Input: part model. Units: mm. Frame: model coordinates. A direction names the side the tool comes from. Round coordinates to 2 decimals unless told otherwise and drop trailing zeros. Loops run counter-clockwise (first coordinate to the right, second up) from the corner with the lowest first, then second, coordinate; pieces in that order, holes last.
1) Section B-B, the plane z = 31. Return loops of the section in (x, y).
2) Access query for faces 5 (the face through (101, -7.5, 19)), 6 (the face through (236.865, 0, 3)), 7 (the face through (101, -19.5, 19)). Directions: +Z, -Z, +X, -X, +Y, -Y. A direction counts if a zero-diameter tool reaches every point of the face in a straight line with its end or side. Return the directions, or none.
3) First-contact query: pin 1 (10 mm diameter, centred on y = -17.5, z = 25, fed in from +X); pin 2 (3 mm diameter, centred on x = -11, y = -34, fed in from +Z); pin 3 (13.5 mm diameter, centred on x = 94, z = 23.5, fed in from -Y); pin 4 (10.5 mm diameter, centred on x = -48.13, y = -32, fed in from +Z). Flat tips, straight axial feed; report the tip coordinate or a pass-through.
4) Section C-C, the plane x = -33. Return loops of the section in (y, z).
5) Section A-A, the plane y = 12. Return loops of the section in (x, z).
6) Draft query along Y for faces 1 (the face through (101, 19.5, 19)), 2 (the face through (28.892, -69.675, 2.958)), 3 (the face through (106.48, 13.42, 22.13)), 4 (the face through (28.065, 38.957, 3.042)). Return one class per face: pulls with the +Y half, pulls with the -Y half, needs draft (parallel to the pull), parting line crosses it, or undercut.
7) Ray query, line 1 along Z through (x, y) = (-45.5, -55); line 2 along Y through (x, z) = (93.5, 18); line 3 along X through (y, z) = (-8, 27). Return the intervals inside material, ascending.
8) Section D-D, the plane x = 213. Return loops of the section in (y, z).
from build123d import *

# Parameters (mm, degrees)
F1_DEPTH  = 6
F2_R      = 60
F3_R      = 40
F4_R      = 300
F8_R      = 10
F10_DEPTH = 12
F9_R      = 10
F11_DEPTH = 12
F12_R     = 6.5
F13_DEPTH = 25


with BuildPart() as f1:
    # F0 (on Top) → F1 (new body)
    with BuildSketch(Plane.XY):
        Polygon((101.865418, 62.004674), (-93.134582, 82.5), (-93.134582, -82.5), (101.865418, -62.004674), (236.865418, -62.004674), (236.865418, 62.004674), align=None)
    extrude(amount=F1_DEPTH)

    # F2
    f2_edges = [f1.edges().sort_by_distance(p)[0] for p in [
        (-93.134582, -82.5, 3),
        (-93.134582, 82.5, 3),
    ]]
    fillet(f2_edges, radius=F2_R)

    # F3
    f3_edges = [f1.edges().sort_by_distance(p)[0] for p in [
        (236.865418, -62.004674, 3),
        (236.865418, 62.004674, 3),
    ]]
    fillet(f3_edges, radius=F3_R)

    # F4
    f4_edges = [f1.edges().sort_by_distance(p)[0] for p in [
        (101.865418, -62.004674, 3),
        (101.865418, 62.004674, 3),
    ]]
    fillet(f4_edges, radius=F4_R)

    # F8 (on offset) → F10 (join)
    with BuildSketch(Plane.XZ.offset(-7.5)):
        with BuildLine():
            Line((151.865418, 6), (116.617663, 44.50449))
            ThreePointArc((116.617663, 44.50449), (101.865418, 51), (87.113173, 44.50449))
            Line((87.113173, 44.50449), (51.865418, 6))
            Line((51.865418, 6), (86.229213, 6))
            Line((86.229213, 6), (151.865418, 6))
        make_face()
        with Locations((101.865418, 31)):
            Circle(F8_R, mode=Mode.SUBTRACT)
    extrude(amount=-F10_DEPTH)

    # F9 (on offset) → F11 (join)
    with BuildSketch(Plane.XZ.offset(7.5)):
        with BuildLine():
            Line((151.865418, 6), (116.617663, 44.50449))
            ThreePointArc((116.617663, 44.50449), (101.865418, 51), (87.113173, 44.50449))
            Line((87.113173, 44.50449), (51.865418, 6))
            Line((51.865418, 6), (86.229213, 6))
            Line((86.229213, 6), (151.865418, 6))
        make_face()
        with Locations((101.865418, 31)):
            Circle(F9_R, mode=Mode.SUBTRACT)
    extrude(amount=F11_DEPTH)

    # F12 (on face) → F13 (cut)
    with BuildSketch(Plane.XY.offset(6)):
        with Locations((200.865418, 31.004674)):
            Circle(F12_R)
        with Locations((200.865418, -31.004674)):
            Circle(F12_R)
        with Locations((21.865418, 37.004674)):
            Circle(F12_R)
        with Locations((-48.134582, 32.004674)):
            Circle(F12_R)
        with Locations((-48.134582, -32.004674)):
            Circle(F12_R)
        with Locations((21.865418, -37.004674)):
            Circle(F12_R)
    extrude(amount=-F13_DEPTH, mode=Mode.SUBTRACT)


solid = f1.part
Final values:
1. outline: (74.75, -19.5) - (91.87, -19.5) - (91.87, -7.5) - (74.75, -7.5) - close; (74.75, 7.5) - (91.87, 7.5) - (91.87, 19.5) - (74.75, 19.5) - close; (111.87, -19.5) - (128.98, -19.5) - (128.98, -7.5) - (111.87, -7.5) - close; (111.87, 7.5) - (128.98, 7.5) - (128.98, 19.5) - (111.87, 19.5) - close
2. face 5: +Z, +X, -X
2. face 6: +Z, -Z, +X, +Y, -Y
2. face 7: +Z, +X, -X, -Y
3. pin 1: stops at x = 139.05
3. pin 2: stops at z = 6
3. pin 3: stops at y = -19.5
3. pin 4: passes through
4. outline: (-75.86, 0) - (75.86, 0) - (75.86, 6) - (-75.86, 6) - close
5. outline: (-93.13, 0) - (236.87, 0) - (236.87, 6) - (151.87, 6) - (116.62, 44.5) arc R20 ccw to (87.11, 44.5) - (51.87, 6) - (-93.13, 6) - close; hole circle Ø20 at (101.87, 31)
6. face 1: pulls with the +Y half
6. face 2: pulls with the -Y half
6. face 3: needs draft
6. face 4: undercut
7. line 1: z = 0 to 6
7. line 2: y = -19.5 to -7.5, 7.5 to 19.5
7. line 3: x = 71.09 to 92.7, 111.03 to 132.64
8. outline: (-58.61, 0) - (58.61, 0) - (58.61, 6) - (-58.61, 6) - close
